Autodesk Fusion 360 part; units mm, degrees
sketch "Sketch1" plane through (0, 0, 0) normal (0, 0, 1) x (1, 0, 0)
  line L0 (0, 0) -> (84, 0)
  line L1 (84, 0) -> (84, 100)
  line L2 (84, 100) -> (0, 100)
  line L3 (0, 100) -> (0, 0)
  dimension "d1" = 84
  dimension "d2" = 100
extrude "Extrude1" add sketch "Sketch1" along normal blind 15
shell "Shell1" thickness 2 removed faces 1 at (28, 66.6667, 0)
sketch "Sketch2" plane through (84, 0, 0) normal (1, 0, 0) x (0, 1, 0)
  line L0 (0, 0) -> (100, 0)
  line L1 (100, 0) -> (100, 15)
  line L2 (100, 15) -> (0, 15)
  line L3 (0, 15) -> (0, 0)
  line L4 (0, 7.5) -> (5, 7.5)
  line L5 (100, 7.5) -> (98.4347, 7.5)
  line L6 (98.4347, 7.5) -> (93.4347, 7.5)
  circle A0 centre (5, 7.5) radius 1.75
  circle A1 centre (93.4347, 7.5) radius 1.75
  line L7 (5, 9.25) -> (93.4347, 9.25)
  line L8 (5, 5.75) -> (93.4347, 5.75)
  dimension "d6" = 5
  dimension "d7" = 5
  dimension "d8" = 3.5
  dimension "d9" = 3.5
extrude "Extrude2" cut sketch "Sketch2" against normal blind 225 contours A0 | A0 A1 L7 L8 | A1
sketch "Sketch3" plane through (0, 0, 15) normal (0, 0, 1) x (-1, 0, 0)
  line L0 (0, -100) -> (0, 0)
  line L1 (0, 0) -> (-84, 0)
  line L2 (-84, 0) -> (-84, -100)
  line L3 (-84, -100) -> (0, -100)
  circle A0 centre (-42, -50) radius 17.5
  dimension "d12" = 35
extrude "Extrude3" cut sketch "Sketch3" against normal blind 30 contours A0
sketch "Sketch4" plane through (0, 0, 15) normal (0, 0, 1) x (-1, 0, 0)
  circle A0 centre (-42, -50) radius 17.5
  line L0 (0, -100) -> (0, 0)
  line L1 (0, 0) -> (-84, 0)
  line L2 (-84, 0) -> (-84, -100)
  line L3 (-84, -100) -> (0, -100)
  line L4 (-42, 0) -> (-42, -10)
  line L5 (-42, 0) -> (-58.1, 0)
  line L6 (-58.1, 0) -> (-58.1, -11.8)
  line L7 (-58.1, -11.8) -> (-25.9, -11.8)
  line L8 (-25.9, -11.8) -> (-25.9, 0)
  line L9 (-25.9, 0) -> (-30.9, 0)
  line L10 (-30.9, 0) -> (-30.9, -11.8)
  line L11 (-58.1, 0) -> (-58.1, -11.8)
  line L12 (-58.1, -11.8) -> (-53.1, -11.8)
  line L13 (-53.1, -11.8) -> (-53.1, 0)
  dimension "d15" = 16.1
  dimension "d16" = 11.8
  dimension "d17" = 32.2
  dimension "d18" = 5
  dimension "d19" = 5
extrude "Extrude4" add sketch "Sketch4" along normal blind 17 contours L1 L7 L8 L9 L10 | L1 L5 L6 L7 L11 L12 L13
sketch "Sketch5" plane through (0, 0, 32) normal (0, 0, 1) x (-1, 0, 0)
  line L0 (-30.9, 0) -> (-30.9, -11.8)
  line L1 (-30.9, -11.8) -> (-25.9, -11.8)
  line L2 (-25.9, -11.8) -> (-25.9, 0)
  line L3 (-25.9, 0) -> (-30.9, 0)
  circle A0 centre (-28.4, -5.9) radius 1.5
  dimension "d22" = 3
sketch "Sketch6" plane through (0, 0, 32) normal (0, 0, 1) x (-1, 0, 0)
  line L0 (-53.1, -11.8) -> (-53.1, 0)
  line L1 (-53.1, 0) -> (-58.1, 0)
  line L2 (-58.1, 0) -> (-58.1, -11.8)
  line L3 (-58.1, -11.8) -> (-53.1, -11.8)
  circle A0 centre (-55.6, -5.9) radius 1.5
  dimension "d23" = 3
extrude "Extrude5" cut sketch "Sketch6" sketch "Sketch5" against normal blind 12 contours A0 of sketch 2 contours A0
sketch "Sketch7" plane through (30.9, 0, 0) normal (1, 0, 0) x (0, 1, 0)
  line L0 (0, 15) -> (11.8, 15)
  line L1 (11.8, 15) -> (11.8, 32)
  line L2 (11.8, 32) -> (0, 32)
  line L3 (0, 32) -> (0, 15)
  line L4 (8.4, 27.7438) -> (3.4, 27.7438)
  line L5 (3.4, 27.7438) -> (3.4, 25.7438)
  line L6 (3.4, 25.7438) -> (8.4, 25.7438)
  line L7 (8.4, 25.7438) -> (8.4, 27.7438)
  line L8 (8.4, 27.7438) -> (3.4, 25.7438) construction
  line L9 (3.4, 27.7438) -> (8.4, 25.7438) construction
  point P0 (5.9, 26.7438)
  dimension "d26" = 5
  dimension "d27" = 2
extrude "Extrude6" cut sketch "Sketch7" along normal blind -5 and the other way blind -34 contours L4 L5 L6 L7
Can you work these out from the model? Positions are in its coordinate system, mm. A direction names the side the tool comes from. Round coordinates to 2 decimals unless told otherwise and drop trailing zeros. Order: outer loops, then holes, each group sorted by start corner. A loop starts at its lowest first (then second) coordinate and runs counter-clockwise, first axis right, second up. Notation, with made-up numbers: (-23.5, -3.75) -> (-5.5, -3.75) arc R6 cw to (-5.5, 0.25) -> close; hole circle Ø7 at (65.5, 48). An arc over 180 degrees is marked (long way). Return JSON: item names as keys, results as strings. Group by question number.
1. I need wall thicknesses on line 1 (X direction, y = 5.9, z = 23.5); line 2 (Y direction, x = 55.6, z = 29.2); line 3 (X direction, y = 65.5, z = 10). Which ranges of each line are inside material? Lowest first, please. Write a range as [from, to].
2. We'd pull the mould along Y, two halves only. Please class faces 6 (the face through (53.1, 6, 23)), 7 (the face through (56, 11.8, 23)), 8 (the face through (82, 49, 5)): released by +Y, released by -Y, zero draft, split by the parting line, or undercut.
3. If we section it at C-C, the plane x = 42: Write out the boundary of the cut face in (y, z), then the cut area to 3 significant figures.
4. Will these pins go through, and if not, where does the flat tip stop? pin 1 (8 mm diameter, centred on x = 32.5, y = 65.5, fed in from +Z); pin 2 (2.5 mm diameter, centred on x = 55.6, y = 5.9, fed in from +Z); pin 3 (1 mm diameter, centred on x = 55, z = 27, fed in from +Y); pin 4 (12 mm diameter, centred on y = 51, z = 24, fed in from -X).
5. Which directions (+Z, -Z, +X, -X, +Y, -Y) give clear straight access to the entire face, cutting with the end or side of a thin tool? Please do faces 1 (the face through (2, 51, 5)), 2 (the face through (58.1, 6, 23)), 3 (the face through (84, 49, 4)), 4 (the face through (25.9, 6, 23)), 5 (the face through (28, 6, 20)).
6. If we section it at D-D, the plane z = 10.5: Write out the boundary of the cut face in (x, y).
7. If we section it at B-B, the plane z = 22: Write out the boundary of the cut face in (x, y).
8. If we section it at A-A, the plane y = 64: Write out the boundary of the cut face in (x, z).
Output values:
{
 "1": {"line 1": "[25.9, 26.9], [29.9, 30.9], [53.1, 54.1], [57.1, 58.1]", "line 2": "[0, 4.4], [7.4, 11.8]", "line 3": "[0, 2], [82, 84]"},
 "2": {"face 6": "zero draft", "face 7": "released by +Y", "face 8": "undercut"},
 "3": {"outline": "(0, 0) -> (2, 0) -> (2, 13) -> (32.5, 13) -> (32.5, 15) -> (0, 15) -> close; (67.5, 13) -> (98, 13) -> (98, 0) -> (100, 0) -> (100, 15) -> (67.5, 15) -> close", "area": "182 mm²"},
 "4": {"pin 1": "z = 15", "pin 2": "z = 20", "pin 3": "y = 11.8", "pin 4": "through"},
 "5": {"face 1": "-Z", "face 2": "+Z, +X, +Y, -Y", "face 3": "+Z, -Z, +X, +Y, -Y", "face 4": "+Z, -X, +Y, -Y", "face 5": "+Z"},
 "6": {"outline": "(0, 0) -> (84, 0) -> (84, 100) -> (0, 100) -> close; hole (2, 2) -> (82, 2) -> (82, 98) -> (2, 98) -> close"},
 "7": {"outline": "(25.9, 0) -> (30.9, 0) -> (30.9, 11.8) -> (25.9, 11.8) -> close; (53.1, 0) -> (58.1, 0) -> (58.1, 11.8) -> (53.1, 11.8) -> close; hole circle Ø3 at (28.4, 5.9); hole circle Ø3 at (55.6, 5.9)"},
 "8": {"outline": "(0, 0) -> (2, 0) -> (2, 5.75) -> (0, 5.75) -> close; (0, 9.25) -> (2, 9.25) -> (2, 13) -> (31.5, 13) -> (31.5, 15) -> (0, 15) -> close; (52.5, 13) -> (82, 13) -> (82, 9.25) -> (84, 9.25) -> (84, 15) -> (52.5, 15) -> close; (82, 0) -> (84, 0) -> (84, 5.75) -> (82, 5.75) -> close"}
}
